from build123d import *

# Parameters (mm, degrees)
BOSS_EXTRUDE1_DEPTH = 10
CUT_EXTRUDE1_DEPTH  = 10


with BuildPart() as part:
    # Sketch1 → Boss-Extrude1 (new body)
    with BuildSketch(Plane.XY):
        with BuildLine():
            Line((-1.5, 16.91317157), (-1.5, 12.91317157))
            ThreePointArc((-1.5, 12.91317157), (-3.364647586, 12.557035742), (-5.157547679, 11.933134623))
            Line((-5.157547679, 11.933134623), (-7.157547679, 15.397236238))
            Line((-7.157547679, 15.397236238), (-9.755623891, 13.897236238))
            Line((-9.755623891, 13.897236238), (-7.755623891, 10.433134623))
            ThreePointArc((-7.755623891, 10.433134623), (-9.192388155, 9.192388155), (-10.433134623, 7.755623891))
            Line((-10.433134623, 7.755623891), (-13.897236238, 9.755623891))
            Line((-13.897236238, 9.755623891), (-15.397236238, 7.157547679))
            Line((-15.397236238, 7.157547679), (-11.933134623, 5.157547679))
            ThreePointArc((-11.933134623, 5.157547679), (-12.557035742, 3.364647586), (-12.91317157, 1.5))
            Line((-12.91317157, 1.5), (-16.91317157, 1.5))
            Line((-16.91317157, 1.5), (-16.91317157, -1.5))
            Line((-16.91317157, -1.5), (-12.91317157, -1.5))
            ThreePointArc((-12.91317157, -1.5), (-12.557035742, -3.364647586), (-11.933134623, -5.157547679))
            Line((-11.933134623, -5.157547679), (-15.397236238, -7.157547679))
            Line((-15.397236238, -7.157547679), (-13.897236238, -9.755623891))
            Line((-13.897236238, -9.755623891), (-10.433134623, -7.755623891))
            ThreePointArc((-10.433134623, -7.755623891), (-9.192388155, -9.192388155), (-7.755623891, -10.433134623))
            Line((-7.755623891, -10.433134623), (-9.755623891, -13.897236238))
            Line((-9.755623891, -13.897236238), (-7.157547679, -15.397236238))
            Line((-7.157547679, -15.397236238), (-5.157547679, -11.933134623))
            ThreePointArc((-5.157547679, -11.933134623), (-3.364647586, -12.557035742), (-1.5, -12.91317157))
            Line((-1.5, -12.91317157), (-1.5, -16.91317157))
            Line((-1.5, -16.91317157), (1.5, -16.91317157))
            Line((1.5, -16.91317157), (1.5, -12.91317157))
            ThreePointArc((1.5, -12.91317157), (3.364647586, -12.557035742), (5.157547679, -11.933134623))
            Line((5.157547679, -11.933134623), (7.157547679, -15.397236238))
            Line((7.157547679, -15.397236238), (9.755623891, -13.897236238))
            Line((9.755623891, -13.897236238), (7.755623891, -10.433134623))
            ThreePointArc((7.755623891, -10.433134623), (9.192388155, -9.192388155), (10.433134623, -7.755623891))
            Line((10.433134623, -7.755623891), (13.897236238, -9.755623891))
            Line((13.897236238, -9.755623891), (15.397236238, -7.157547679))
            Line((15.397236238, -7.157547679), (11.933134623, -5.157547679))
            ThreePointArc((11.933134623, -5.157547679), (12.557035742, -3.364647586), (12.91317157, -1.5))
            Line((12.91317157, -1.5), (16.91317157, -1.5))
            Line((16.91317157, -1.5), (16.91317157, 1.5))
            Line((16.91317157, 1.5), (12.91317157, 1.5))
            ThreePointArc((12.91317157, 1.5), (12.557035742, 3.364647586), (11.933134623, 5.157547679))
            Line((11.933134623, 5.157547679), (15.397236238, 7.157547679))
            Line((15.397236238, 7.157547679), (13.897236238, 9.755623891))
            Line((13.897236238, 9.755623891), (10.433134623, 7.755623891))
            ThreePointArc((10.433134623, 7.755623891), (9.192388155, 9.192388155), (7.755623891, 10.433134623))
            Line((7.755623891, 10.433134623), (9.755623891, 13.897236238))
            Line((9.755623891, 13.897236238), (7.157547679, 15.397236238))
            Line((7.157547679, 15.397236238), (5.157547679, 11.933134623))
            ThreePointArc((5.157547679, 11.933134623), (3.364647586, 12.557035742), (1.5, 12.91317157))
            Line((1.5, 12.91317157), (1.5, 16.91317157))
            Line((1.5, 16.91317157), (-1.5, 16.91317157))
        make_face()
    extrude(amount=BOSS_EXTRUDE1_DEPTH)

    # Sketch2 → Cut-Extrude1 (cut)
    with BuildSketch(Plane.XY.offset(10)):
        with BuildLine():
            Line((2.562713194, -0.438749457), (0.901388421, 2.438749457))
            ThreePointArc((0.901388421, 2.438749457), (-2.25166605, -1.3), (2.562713194, -0.438749457))
        make_face()
    extrude(amount=-CUT_EXTRUDE1_DEPTH, mode=Mode.SUBTRACT)


solid = part.part
For this review, take the finished solid that the model builds, in its own axes (mm). A direction names the side the tool comes from. Round coordinates to 2 decimals unless told otherwise and drop trailing zeros. Loops run counter-clockwise (first coordinate to the right, second up) from the corner with the lowest first, then second, coordinate; pieces in that order, holes last. Notation, with made-up numbers: (-14.5, 75) - (18.5, 75) arc R12 cw to (18.5, 81) - close; hole circle Ø2 at (25, 77). An arc over 180 degrees is marked (long way). One line per question, with ' | ' between items.
Q1. Tool access review of faces 1 (the flat face through (8.77, -12.19, 4.93)), 2 (the flat face through (-8.74, -12.14, 4.93)), 3 (the cylindrical face through (-9.211, -9.174, 4.93)), 4 (the flat face through (-6.17, -13.69, 4.93)): name each direction out of +Z, -Z, +X, -X, +Y, -Y from which nothing blocks a thin tool from reaching the whole face with its end or side.
Taken from the geometry:
face 1: +Z, -Z, +X | face 2: +Z, -Z, -X | face 3: +Z, -Z | face 4: +Z, -Z, -Y
Q2. The part is to be moulded in two halves that separate along Y. For faces 5 (the flat face through (6.17, 13.69, 4.93)), 6 (the flat face through (15, 1.5, 5)), 7 (the flat face through (-13.641, -6.144, 4.93)), 8 (the flat face through (0, -16.913, 5)), say which applies: released by +Y, released by -Y, zero draft, split by the parting line, or undercut.
Taken from the geometry:
face 5: released by +Y | face 6: undercut | face 7: undercut | face 8: released by -Y
Q3. Take a section at C-C (x = -8.5). Give the boundary of the cut face in (y, z).
Taken from the geometry:
outline: (-14.62, 0) - (-11.72, 0) - (-11.72, 10) - (-14.62, 10) - close; (-9.84, 0) - (9.84, 0) - (9.84, 10) - (-9.84, 10) - close; (11.72, 0) - (14.62, 0) - (14.62, 10) - (11.72, 10) - close
Q4. Take a section at B-B (y = -1). Give the boundary of the cut face in (x, z), and give its area (3 significant figures).
Taken from the geometry:
outline: (-16.91, 0) - (-2.4, 0) - (-2.4, 10) - (-16.91, 10) - close; (2.4, 0) - (16.91, 0) - (16.91, 10) - (2.4, 10) - close | area: 290 mm²
Q5. For pin 1 (12 mm diameter, centred on x = -10.5, y = -2.5, fed in from -Z); pin 2 (1 mm diameter, centred on x = 7.5, z = 2.5, fed in from +Y); pin 3 (4.5 mm diameter, centred on x = 15, z = 3.5, fed in from -Y); pin 4 (1.2 mm diameter, centred on x = -15, z = 3, fed in from -Y), all flat-tipped, find the tip position at first contact; note any pin that passes through.
Taken from the geometry:
pin 1: stops at z = 0 | pin 2: stops at y = 15.4 | pin 3: stops at y = -9.76 | pin 4: stops at y = -8.88
Q6. Take a section at D-D (x = 12.5). Give the boundary of the cut face in (y, z).
Taken from the geometry:
outline: (-8.95, 0) - (-5.48, 0) - (-5.48, 10) - (-8.95, 10) - close; (-3.57, 0) - (3.57, 0) - (3.57, 10) - (-3.57, 10) - close; (5.48, 0) - (8.95, 0) - (8.95, 10) - (5.48, 10) - close
Q7. Take a section at A-A (x = 0). Give the boundary of the cut face in (y, z).
Taken from the geometry:
outline: (-16.91, 0) - (-2.6, 0) - (-2.6, 10) - (-16.91, 10) - close; (2.6, 0) - (16.91, 0) - (16.91, 10) - (2.6, 10) - close
Q8. For line 1 along Y through (x, z) = (0, 3.75); line 2 along Y through (x, z) = (-13.5, 1.5); line 3 along X through (y, z) = (8, 5.75), list the stretches that pass through material, from the lowest coordinate up. Write a range as [from, to].
Taken from the geometry:
line 1: y = [-16.91, -2.6], [2.6, 16.91] | line 2: y = [-9.53, -6.06], [-1.5, 1.5], [6.06, 9.53] | line 3: x = [-14.91, -10.86], [-10.25, 10.25], [10.86, 14.91]
